```python
from build123d import *

# Parameters (mm, degrees)
SKETCH_1_R      = 1.6
EXTRUDE_1_DEPTH = 3


with BuildPart() as part:
    # 草图1 → 凸台-拉伸1 (new body)
    with BuildSketch(Plane.XY):
        with BuildLine():
            Line((0, -52), (77, -52))
            ThreePointArc((77, -52), (79.121320344, -51.121320344), (80, -49))
            Line((80, -49), (80, 0))
            ThreePointArc((80, 0), (79.121320344, 2.121320344), (77, 3))
            Line((77, 3), (0, 3))
            ThreePointArc((0, 3), (-2.121320344, 2.121320344), (-3, 0))
            Line((-3, 0), (-3, -49))
            ThreePointArc((-3, -49), (-2.121320344, -51.121320344), (0, -52))
        make_face()
        Circle(SKETCH_1_R, mode=Mode.SUBTRACT)
        with Locations((77, 0)):
            Circle(SKETCH_1_R, mode=Mode.SUBTRACT)
        with Locations((0, -49)):
            Circle(SKETCH_1_R, mode=Mode.SUBTRACT)
        with Locations((77, -49)):
            Circle(SKETCH_1_R, mode=Mode.SUBTRACT)
        with BuildLine():
            Line((16.5, -41.5), (60.5, -41.5))
            ThreePointArc((60.5, -41.5), (62.621320344, -40.621320344), (63.5, -38.5))
            Line((63.5, -38.5), (63.5, -10.5))
            ThreePointArc((63.5, -10.5), (62.621320344, -8.378679656), (60.5, -7.5))
            Line((60.5, -7.5), (16.5, -7.5))
            ThreePointArc((16.5, -7.5), (14.378679656, -8.378679656), (13.5, -10.5))
            Line((13.5, -10.5), (13.5, -38.5))
            ThreePointArc((13.5, -38.5), (14.378679656, -40.621320344), (16.5, -41.5))
        make_face(mode=Mode.SUBTRACT)
    extrude(amount=EXTRUDE_1_DEPTH)


solid = part.part
```
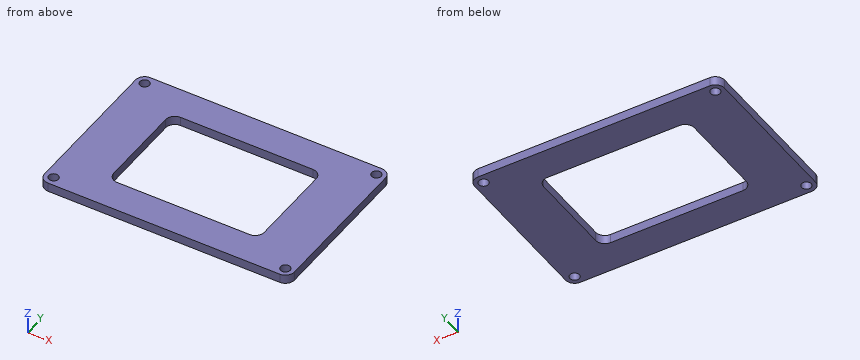
Model file for the job. Use its own axes, mm. Coordinates: 2 decimals unless noted, no trailing zeros. Write each loop counter-clockwise with the first axis right and the second up, starting at its lowest first coordinate (ties: lowest second). Pieces come first, ordered by that corner, then holes. Notation, with made-up numbers: (9, 46) - (24, 46) arc R15 ccw to (24, 62) - close; hole circle Ø5 at (-29, 63.25). An arc over 180 degrees is marked (long way). Use a Markdown table: item, result. Add a question column.
Item 1: Band-saw the part on A-A, the plane x = 51.5. Write the cut outline in (y, z).
Item 2: Drill centre lines: line 1 along Y through (x, z) = (0, 1.8); line 2 along X through (y, z) = (-34.5, 0.1); line 3 along Y through (x, z) = (37.5, 1.7). Where is each one in solid material? Low to high.
Item 3: Band-saw the part on C-C, the plane z = 1.4. Write the cut outline in (x, y).
Item 4: Band-saw the part on B-B, the plane y = -15. Write the cut outline in (x, z), and give its area (3 significant figures).
A:
| question | item | result |
|---|---|---|
| 1 | outline | (-52, 0) - (-41.5, 0) - (-41.5, 3) - (-52, 3) - close; (-7.5, 0) - (3, 0) - (3, 3) - (-7.5, 3) - close |
| 2 | line 1 | y = -52 to -50.6, -47.4 to -1.6, 1.6 to 3 |
| 2 | line 2 | x = -3 to 13.5, 63.5 to 80 |
| 2 | line 3 | y = -52 to -41.5, -7.5 to 3 |
| 3 | outline | (-3, -49) arc R3 ccw to (0, -52) - (77, -52) arc R3 ccw to (80, -49) - (80, 0) arc R3 ccw to (77, 3) - (0, 3) arc R3 ccw to (-3, 0) - close; hole circle Ø3.2 at (0, -49); hole circle Ø3.2 at (0, 0); hole (13.5, -38.5) arc R3 ccw to (16.5, -41.5) - (60.5, -41.5) arc R3 ccw to (63.5, -38.5) - (63.5, -10.5) arc R3 ccw to (60.5, -7.5) - (16.5, -7.5) arc R3 ccw to (13.5, -10.5) - close; hole circle Ø3.2 at (77, -49); hole circle Ø3.2 at (77, 0) |
| 4 | outline | (-3, 0) - (13.5, 0) - (13.5, 3) - (-3, 3) - close; (63.5, 0) - (80, 0) - (80, 3) - (63.5, 3) - close |
| 4 | area | 99.0 mm² |
